The figure shows three views and two pictorial views of one solid part (mm, origin at its lowest corner). Answer the questions. A direction names the side the tool comes from. Coordinates: 2 decimals unless noted, no trailing zeros. Write each loop counter-clockwise with the first axis right and the second up, starting at its lowest first coordinate (ties: lowest second). Pieces come first, ordered by that corner, then holes. Notation, with made-up numbers: M 62,81 L 95,81 A31 ccw 95,110 Z; hole C -31.75,13 d3. An arc over 180 degrees is marked long. Write item = value, one per line.
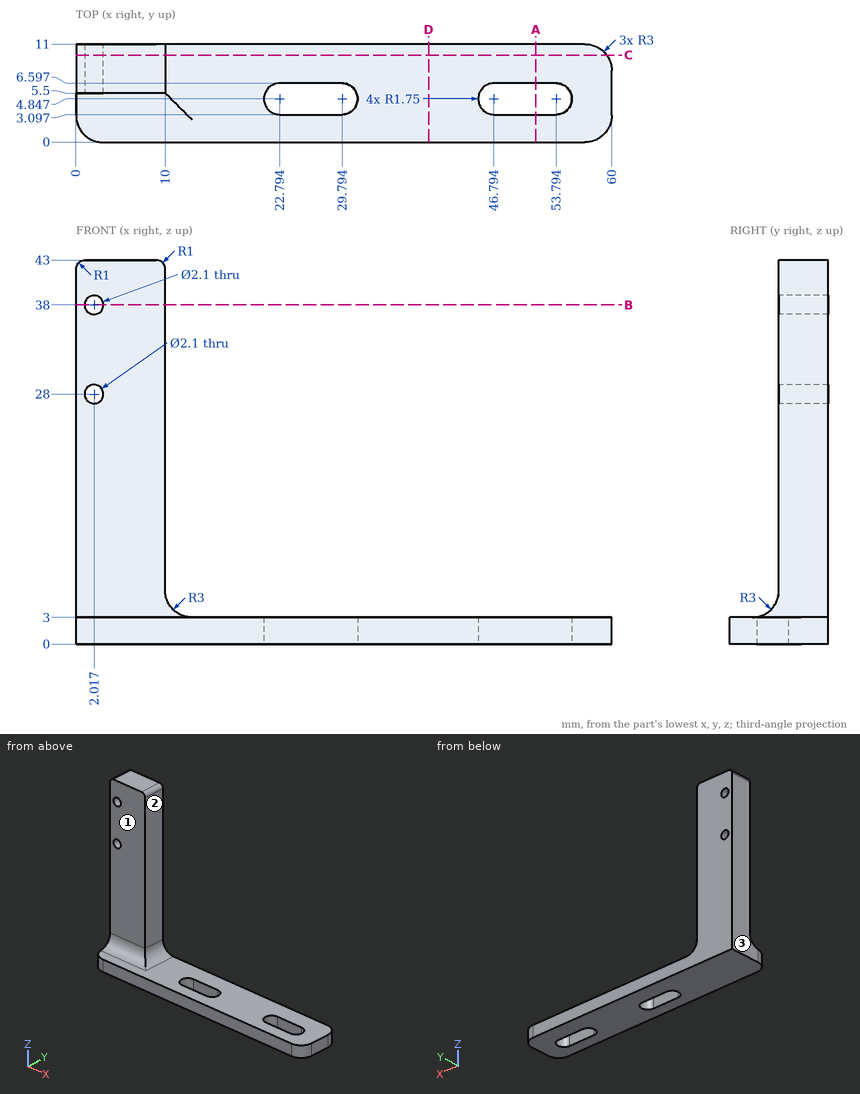
Item 1: Find section B-B (z = 38). Determine the outline of the cut face in (x, y).
Worked answers:
outline = M 0,5.5 L 0.97,5.5 L 0.97,11 L 0,11 Z; M 3.07,5.5 L 10,5.5 L 10,11 L 3.07,11 Z
Item 2: Flat-ended cylindrical pins translate along their axes: pin 1 (8 mm diameter, centred on x = 4.5, z = 19, fed in from -Y); pin 2 (3 mm diameter, centred on y = 8.5, z = 24, fed in from +X); pin 3 (6 mm diameter, centred on x = 19, y = 4, fed in from +Z). Find the tip coordinate at first contact, or state that the pin passes through.
Worked answers:
pin_1 = 5.5
pin_2 = 10
pin_3 = 3
Item 3: Consider line 1 along Z through (x, y) = (19.5, 1); line 2 along X through (y, z) = (7, 18); line 3 along Z through (x, y) = (2.5, 3.25) (1 decimal). Determine where each line is inside the solid, lowest interval first. Write a range as from..to.
Worked answers:
line_1 = 0..3
line_2 = 0..10
line_3 = 0..3.1
Item 4: Which of the six approach directions +Z, -Z, +X, -X, +Y, -Y give full straight-line access (tool end or side, diameter ignored) to the marked faces 1, 2 and 3?
Worked answers:
face_1 = +Z, +X, -X, -Y
face_2 = +Z, +X, +Y, -Y
face_3 = +Z, -Z, -X, +Y, -Y
Item 5: Find section A-A (x = 51.5). Determine the outline of the cut face in (y, z).
Worked answers:
outline = M 0,0 L 3.1,0 L 3.1,3 L 0,3 Z; M 6.6,0 L 11,0 L 11,3 L 6.6,3 Z
Item 6: Find section D-D (x = 39.5). Determine the outline of the cut face in (y, z).
Worked answers:
outline = M 0,0 L 11,0 L 11,3 L 0,3 Z
Item 7: Find section C-C (y = 9.75). Determine the outline of the cut face in (x, z), and give its area (3 significant figures).
Worked answers:
outline = M 0,0 L 59.44,0 L 59.44,3 L 13,3 A3 cw 10,6 L 10,42 A1 ccw 9,43 L 1,43 A1 ccw 0,42 Z; hole C 2.02,28 d2.1; hole C 2.02,38 d2.1
area = 573 mm²
